```python
from build123d import *

# Parameters (mm, degrees)
F0_W      = 127
F0_H      = 99.441
F1_DEPTH  = 18.415
F2_W      = 18.5674
F2_H      = 30.734
F3_DEPTH  = 88.9
F7_R      = 6.223
F8_DEPTH  = 31.75
F10_R     = 6.223
F11_DEPTH = 31.75
F9_R      = 3.175
F12_DEPTH = 31.75


with BuildPart() as f1:
    # F0 (on Top) → F1 (new body)
    with BuildSketch(Plane.XY):
        with Locations((63.5, 49.7205)):
            Rectangle(F0_W, F0_H)
    extrude(amount=F1_DEPTH)

    # F2 (on Top) → F3 (join)
    with BuildSketch(Plane.XY):
        with Locations((-9.2837, 56.007)):
            Rectangle(F2_W, F2_H)
    extrude(amount=F3_DEPTH)

    # F5 (on offset) → F6 (revolve)
    with BuildSketch(Plane.XZ.offset(-56.007)):
        Polygon((0, 66.04), (0, 59.69), (10.033, 59.69), (10.033, 62.0395), (3.175, 66.04), align=None)
    revolve(axis=Axis((5.0165, 56.007, 59.69), (1, 0, 0)))

    # F7 (on face) → F8 (join)
    with BuildSketch(Plane.XY.offset(18.415)):
        with Locations((95.25, 12.7)):
            Circle(F7_R)
        with Locations((101.6, 27.686)):
            Circle(F7_R)
        with Locations((101.6, 65.786)):
            Circle(F7_R)
        with Locations((28.575, 56.007)):
            Circle(F7_R)
        with Locations((28.575, 31.75)):
            Circle(F7_R)
    extrude(amount=F8_DEPTH)

    # F10 (on face) → F11 (join)
    with BuildSketch(Plane.XY.offset(50.165)):
        with Locations((95.25, 12.7)):
            Circle(F10_R)
        with Locations((28.575, 31.75)):
            Circle(F10_R)
    extrude(amount=F11_DEPTH)

    # F9 (on face) → F12 (cut)
    with BuildSketch(Plane.XY.offset(50.165)):
        with Locations((28.575, 56.007)):
            Circle(F9_R)
        with Locations((101.6, 65.786)):
            Circle(F9_R)
        with Locations((101.6, 27.686)):
            Circle(F9_R)
    extrude(amount=-F12_DEPTH, mode=Mode.SUBTRACT)


solid = f1.part
```
Part model, mm, in its own coordinate system. A direction names the side the tool comes from. Give positions to 0.01 mm unless a question says otherwise; leave off trailing zeros. Order: outer loops, then holes, each group sorted by start corner. A loop starts at its lowest first (then second) coordinate and runs counter-clockwise, first axis right, second up. Notation, with made-up numbers: M -16,-20.75 L 29,-20.75 A18 cw 29,10.25 Z; hole C 43,55 d8. An arc over 180 degrees is marked long. Use a Markdown table: item, result. Add a question column.
(1) Saw through at D-D, the plane x = 84.5. Give the cut face in (y, z) (3 decimals), and give its area (3 significant figures).
(2) Saw through at C-C, the plane y = 14.5. Give the cut face in (x, z) (3 decimals).
(3) 3-axis set-ups, long thin cutter, end or side, ignore diameter. For faces 1 (the face through (63, 0, 9)), 2 (the face through (1.57, 49.71, 58.86)), 3 (the face through (27, 59, 50.165)), 4 (the face through (99.08, 63.854, 34.512)), 5 (the face through (10.033, 56, 60)): which of +Z, -Z, +X, -X, +Y, -Y reach the whole face in a straight line?
(4) Mould opens along X. For faces 6 (the face through (0, 20, 9)), 7 (the face through (-9, 56, 88.9)), 8 (the face through (27.887, 52.908, 34.512)), 9 (the face through (101.187, 30.834, 34.512)) say: +X half, -X half, draft (parallel to the pull), parting line (faces both ways), or undercut.
(5) Probe line 1 along Y through (x, z) = (101.6, 25); line 2 along Y through (x, z) = (29, 72); line 3 along Z through (x, y) = (68.5, 51) (3 decimals). List the from-to ranges inside material, lowest first. Write a range as [from, to].
(6) Saw through at A-A, the plane z = 59.69. Give the number of separate pieces and of enclosed holes in the cut face, and give its area (3 significant figures).
(7) Drop flat-ended pins along their axis: P1, Ø4, axis at y = 55.5, z = 59, coming from the +X side; P2, Ø6, axis at x = 107, y = 82.5, coming from the +Z side (3 decimals); P3, Ø13.5, axis at x = 101, y = 63.5, coming from the +Z side (3 decimals); P4, Ø8, axis at x = 112, z = 40.5, coming from the -Y side. Give the stop position or say it passes through.
Answer key:
| question | item | result |
|---|---|---|
| 1 | outline | M 0,0 L 99.441,0 L 99.441,18.415 L 0,18.415 Z |
| 1 | area | 1,830 mm^2 |
| 2 | outline | M 0,0 L 127,0 L 127,18.415 L 101.207,18.415 L 101.207,81.915 L 89.293,81.915 L 89.293,18.415 L 0,18.415 Z |
| 3 | face 1 | +Z, -Z, +X, -X, -Y |
| 3 | face 2 | +X |
| 3 | face 3 | +Z, +X, +Y |
| 3 | face 4 | +Z |
| 3 | face 5 | +Z, +X, +Y, -Y |
| 4 | face 6 | -X half |
| 4 | face 7 | draft |
| 4 | face 8 | undercut |
| 4 | face 9 | undercut |
| 5 | line 1 | [21.46, 24.51], [30.86, 33.91], [59.56, 62.61], [68.96, 72.01] |
| 5 | line 2 | [25.54, 37.96] |
| 5 | line 3 | [0, 18.415] |
| 6 | separate pieces | 3 |
| 6 | enclosed holes | 0 |
| 6 | area | 914 mm^2 |
| 7 | P1 | x = 10.03 |
| 7 | P2 | z = 18.415 |
| 7 | P3 | z = 50.165 |
| 7 | P4 | through |
